Check sheet for the modelled part. Datum: model origin and axes. Units: mm. A direction names the side the tool comes from. Give positions to 0.01 mm unless a question says otherwise; leave off trailing zeros. Loops run counter-clockwise (first coordinate to the right, second up) from the corner with the lowest first, then second, coordinate; pieces in that order, holes last. Notation, with made-up numbers: M -12,34 L 11,34 A26 ccw 11,65 Z; hole C -31.75,27.5 d7. An arc over 180 degrees is marked long. One line per question, with ' | ' between items. Start each with the question number.
from build123d import *

# Parameters (mm, degrees)
SKETCH1_W             = 110
SKETCH1_H             = 78
BOSS_EXTRUDE1_DEPTH   = 36
M3_TAPPED_HOLE2_D     = 2.5
M3_TAPPED_HOLE2_DEPTH = 5
M3_TAPPED_HOLE2_TIP   = 0.751075774
SKETCH8_W             = 16
SKETCH8_H             = 77
CUT_EXTRUDE2_DEPTH    = 35
F_3_0MM_DOWEL_HOLE1_D = 3
SKETCH12_W            = 10
SKETCH12_H            = 67
CUT_EXTRUDE4_DEPTH    = 25
SKETCH13_W            = 10
SKETCH13_H            = 10
CUT_EXTRUDE5_DEPTH    = 35
CUT_EXTRUDE7_DEPTH    = 67
CUT_EXTRUDE8_DEPTH    = 2
M3_TAPPED_HOLE3_D     = 2.5
FILLET1_R             = 2
CUT_EXTRUDE9_DEPTH    = 37


with BuildPart() as part:
    # Sketch1 → Boss-Extrude1 (new body)
    with BuildSketch(Plane(origin=(0, 0, 0), x_dir=(1, 0, 0), z_dir=(0, 1, 0))):
        with Locations((55, 39)):
            Rectangle(SKETCH1_W, SKETCH1_H)
    extrude(amount=BOSS_EXTRUDE1_DEPTH)

    # M3 Tapped Hole2
    with Locations(Plane(origin=(0, 0, 0), x_dir=(-1, 0, 0), z_dir=(0, -1, 0))):
        with Locations((-67.5, 25), (-67.5, 52.5), (-31.5, 52.5)):
            Hole(M3_TAPPED_HOLE2_D / 2, depth=M3_TAPPED_HOLE2_DEPTH)
            with Locations((0, 0, -(M3_TAPPED_HOLE2_DEPTH + M3_TAPPED_HOLE2_TIP / 2))):  # 118° drill point
                Cone(0, M3_TAPPED_HOLE2_D / 2, M3_TAPPED_HOLE2_TIP, mode=Mode.SUBTRACT)

    # Sketch8 → Cut-Extrude2 (cut)
    with BuildSketch(Plane(origin=(0, 36, 0), x_dir=(1, 0, 0), z_dir=(0, 1, 0))):
        with Locations((8, 39.5)):
            Rectangle(SKETCH8_W, SKETCH8_H)
    extrude(amount=-CUT_EXTRUDE2_DEPTH, mode=Mode.SUBTRACT)

    # Ø3.0mm Dowel Hole1 (through all)
    with Locations(Plane(origin=(0, 0, 0), x_dir=(-1, 0, 0), z_dir=(0, -1, 0))):
        with Locations((-5, 4)):
            Hole(F_3_0MM_DOWEL_HOLE1_D / 2)

    # Sketch12 → Cut-Extrude4 (cut)
    with BuildSketch(Plane(origin=(0, 36, 0), x_dir=(1, 0, 0), z_dir=(0, 1, 0))):
        with Locations((105, 34.5)):
            Rectangle(SKETCH12_W, SKETCH12_H)
    extrude(amount=-CUT_EXTRUDE4_DEPTH, mode=Mode.SUBTRACT)

    # Sketch13 → Cut-Extrude5 (cut)
    with BuildSketch(Plane(origin=(0, 36, 0), x_dir=(1, 0, 0), z_dir=(0, 1, 0))):
        with Locations((105, 73)):
            Rectangle(SKETCH13_W, SKETCH13_H)
    extrude(amount=-CUT_EXTRUDE5_DEPTH, mode=Mode.SUBTRACT)

    # Sketch15 → Cut-Extrude7 (cut)
    with BuildSketch(Plane(origin=(0, 0, -68), x_dir=(-1, 0, 0), z_dir=(0, 0, -1))):
        Polygon((-110, 6), (-100, 11), (-110, 11), align=None)
    extrude(amount=-CUT_EXTRUDE7_DEPTH, mode=Mode.SUBTRACT)

    # Sketch16 → Cut-Extrude8 (cut, through all)
    with BuildSketch(Plane(origin=(0, 0, -1), x_dir=(-1, 0, 0), z_dir=(0, 0, -1))):
        with BuildLine():
            Line((-115, 30.09689573), (-105, 30.09689573))
            ThreePointArc((-105, 30.09689573), (-103, 28.09689573), (-105, 26.09689573))
            Line((-105, 26.09689573), (-115, 26.09689573))
            ThreePointArc((-115, 26.09689573), (-117, 28.09689573), (-115, 30.09689573))
        make_face()
    extrude(amount=-CUT_EXTRUDE8_DEPTH, mode=Mode.SUBTRACT)

    # M3 Tapped Hole3 (through all)
    with Locations(Plane.XY):
        with Locations((10, 17.5)):
            Hole(M3_TAPPED_HOLE3_D / 2)

    # Fillet1
    fillet1_edges = [part.edges().sort_by_distance(p)[0] for p in [
        (110, 36, -0.5),
        (0, 36, -0.5),
        (0, 0.5, -78),
        (110, 0.5, -78),
    ]]
    fillet(fillet1_edges, radius=FILLET1_R)

    # Sketch20 → Cut-Extrude9 (cut, through all)
    with BuildSketch(Plane(origin=(0, 0, 0), x_dir=(-1, 0, 0), z_dir=(0, -1, 0))):
        with BuildLine():
            Line((-102, 72), (-113.136440261, 72))
            ThreePointArc((-113.136440261, 72), (-115.136440261, 74), (-113.136440261, 76))
            Line((-113.136440261, 76), (-102, 76))
            ThreePointArc((-102, 76), (-100, 74), (-102, 72))
        make_face()
    extrude(amount=-CUT_EXTRUDE9_DEPTH, mode=Mode.SUBTRACT)


solid = part.part
Q1. Material ranges on probe 1 along X at (y, z) = (3.9, -52.5); probe 2 along X at (y, z) = (3.65, -25); probe 3 along Z at (x, y) = (67.5, 2.9), recorded low to high. Write a range as from..to.
Q2. Cross-section at B-B (z = -4). Record the cut outline in (x, y), and give its area (3 significant figures).
Q3. Draft check along X on faces 1 (the flat face through (54, 18, -78)), 2 (the flat face through (110, 3, -36)), 3 (the conical face through (31.4, 5.62, -52.31)), 4 (the cylindrical face through (68.69, 2.54, -52.88)). Enter one of: released by +X, released by -X, zero draft, split by the parting line, or undercut.
Q4. Cross-section at C-C (z = -19). Record the cut outline in (x, y).
Q5. Access from +Z, -Z, +X, -X, +Y, -Y to the whole of each face (thin tool, end or side, straight path). Record for faces 5 (the flat face through (54, 0, -40)), 6 (the cylindrical face through (11.25, 17.55, -0.51)), 7 (the flat face through (105, 21, -1)), 8 (the flat face through (8, 19, -1)), 9 (the cylindrical face through (31.34, 2.54, -53.74)).
Q6. Cross-section at A-A (x = 5). Record the cut outline in (y, z), and give its area (3 significant figures).
Q7. Depth check by flat-ended pin: P1, Ø2, axis at x = 68.5, y = 25.5, coming from the +Z side; P2, Ø8, axis at x = 105.5, y = 15, coming from the -Z side; P3, Ø1, axis at y = 31, z = -61, coming from the -X side; P4, Ø2, axis at y = 16, z = -21.5, coming from the +X side. Enter the tip coordinate at first touch or a pass-through.
Solved:
1) probe 1: x = 16..30.25, 32.75..66.25, 68.75..110 | probe 2: x = 16..66.25, 68.75..110 | probe 3: z = -78..-53.75, -51.25..-26.25, -23.75..0
2) outline: M 0,0 L 3.5,0 L 3.5,1 L 0,1 Z; M 6.5,0 L 110,0 L 110,6 L 100,11 L 100,36 L 16,36 L 16,1 L 6.5,1 Z | area: 3,120 mm²
3) face 1: zero draft | face 2: released by +X | face 3: undercut | face 4: undercut
4) outline: M 0,0 L 110,0 L 110,6 L 100,11 L 100,36 L 16,36 L 16,1 L 0,1 Z
5) face 5: +Z, -Z, +X, -X, -Y | face 6: +Z, -Z | face 7: -Z, +X, +Y | face 8: -Z, -X, +Y | face 9: -Y
6) outline: M 0,-78 L 1,-78 L 1,-5.5 L 0,-5.5 Z; M 0,-2.5 L 1,-2.5 L 1,-1 L 36,-1 L 36,0 L 0,0 Z | area: 110 mm²
7) P1: stops at z = 0 | P2: stops at z = -1 | P3: stops at x = 16 | P4: stops at x = 100
